Build history of the part. All positions in model axes, mm. A direction names the side the tool comes from. Give positions to 0.01 mm unless a question says otherwise; leave off trailing zeros. Write each loop counter-clockwise with the first axis right and the second up, starting at its lowest first coordinate (ties: lowest second). Pieces come first, ordered by that corner, then holes. Notation, with made-up numbers: (50, 26.5) -> (96, 26.5) arc R12 cw to (96, 49.5) -> close; hole circle Ø9 at (-16, 4). An arc over 180 degrees is marked (long way). Put each result on its own line as item: value. Start each with the question number.
Item 1: Tool access for faces 1 (the flat face through (5.775, -3.397, 3.465)), 2 (the flat face through (5.83, 3.3, 3.46)), 3 (the flat face through (-5.83, -3.3, 3.46)): list every direction of +Z, -Z, +X, -X, +Y, -Y with a clear straight run to the whole face (end or side of a thin tool).
Item 2: Slice it at C-C, the plane y = 6.5. List the corners of the cut face in (x, z), plus the area to 3 significant figures.
Item 3: Slice it at D-D, the plane x = 7.25. List the corners of the cut face in (y, z).
Item 4: Two-plate mould, pull along Y, no slides. Class faces 4 (the cylindrical face through (-1.003, -4.515, 2.958)), 5 (the flat face through (-5.775, 3.397, 3.465)), 6 (the flat face through (0, 7, 1)): pulls with the +Y half, pulls with the -Y half, needs draft (parallel to the pull), parting line crosses it, or undercut.
Item 5: Flat gauge pins, fed straight in: pin 1 Ø1 at (y, z) = (1, 5.5) entering from -X; pin 2 Ø1.5 at (x, z) = (2.5, 2.5) entering from -Y; pin 3 Ø3 at (y, z) = (4, 3.5) entering from +X; pin 4 Ø1 at (x, y) = (1, 3.5) entering from +Z. Where does each tip first touch, or does it go through?
Item 6: Slice it at B-B, the plane x = 0. List the corners of the cut face in (y, z) (3 decimals), plus the area to 3 significant figures.
Item 7: Drill centre lines: line 1 along Y through (x, z) = (0, 2.7) (3 decimals); line 2 along Z through (x, y) = (6.5, -4.25); line 3 along Y through (x, z) = (3.75, 3.6). Where is each one in solid material? Low to high.
```python
from build123d import *

# Parameters (mm, degrees)
PAD001_DEPTH      = 6
SKETCH004_R       = 8.4
PAD002_DEPTH      = 1
SKETCH005_R       = 4.625
POCKET_DEPTH      = 0.001
POCKET_DEPTH_BACK = 6.001


with BuildPart() as part:
    # Sketch003 → Pad001 (new body)
    with BuildSketch(Plane.XY):
        Polygon((7.736494, 0), (3.868247, 6.7), (-3.868247, 6.7), (-7.736494, 0), (-3.868247, -6.7), (3.868247, -6.7), align=None)
    extrude(amount=PAD001_DEPTH)

    # Sketch004 → Pad002 (join)
    with BuildSketch(Plane.XY):
        Circle(SKETCH004_R)
    extrude(amount=PAD002_DEPTH)

    # Sketch005 → Pocket (cut, two sides)
    with BuildSketch(Plane.XY) as pocket_sk:
        Circle(SKETCH005_R)
    extrude(amount=-POCKET_DEPTH, mode=Mode.SUBTRACT)
    extrude(pocket_sk.sketch, amount=POCKET_DEPTH_BACK, mode=Mode.SUBTRACT)


solid = part.part
```
Values follow:
1. face 1: +Z, +X, -Y
1. face 2: +Z, +X, +Y
1. face 3: +Z, -X, -Y
2. outline: (-5.32, 0) -> (5.32, 0) -> (5.32, 1) -> (3.98, 1) -> (3.98, 6) -> (-3.98, 6) -> (-3.98, 1) -> (-5.32, 1) -> close
2. area: 50.5 mm2
3. outline: (-4.24, 0) -> (4.24, 0) -> (4.24, 1) -> (0.84, 1) -> (0.84, 6) -> (-0.84, 6) -> (-0.84, 1) -> (-4.24, 1) -> close
4. face 4: undercut
4. face 5: pulls with the +Y half
4. face 6: needs draft
5. pin 1: x = -7.45
5. pin 2: y = -6.7
5. pin 3: x = 6.29
5. pin 4: through
6. outline: (-8.4, 0) -> (-4.625, 0) -> (-4.625, 6) -> (-6.7, 6) -> (-6.7, 1) -> (-8.4, 1) -> close; (4.625, 0) -> (8.4, 0) -> (8.4, 1) -> (6.7, 1) -> (6.7, 6) -> (4.625, 6) -> close
6. area: 28.3 mm2
7. line 1: -6.7 to -4.625, 4.625 to 6.7
7. line 2: 0 to 1
7. line 3: -6.7 to -2.71, 2.71 to 6.7
